```python
from build123d import *

# Parameters (mm, degrees)
SKETCH2_R           = 22.25
SKETCH2_R_2         = 2.5
BOSS_EXTRUDE1_DEPTH = 2.4
SKETCH3_R           = 12.4
BOSS_EXTRUDE2_DEPTH = 47.3
SKETCH4_R           = 3.25
BOSS_EXTRUDE3_DEPTH = 4
SKETCH5_R           = 2.5
BOSS_EXTRUDE4_DEPTH = 8.4
SKETCH6_R           = 12.385
BOSS_EXTRUDE5_DEPTH = 5.1
SKETCH7_R           = 5.9
BOSS_EXTRUDE6_DEPTH = 7.2


with BuildPart() as part:
    # Sketch2 → Boss-Extrude1 (new body)
    with BuildSketch(Plane(origin=(0, 0, 0), x_dir=(1, 0, 0), z_dir=(0, 1, 0))):
        Circle(SKETCH2_R)
        with Locations((0, 17.45)):
            Circle(SKETCH2_R_2, mode=Mode.SUBTRACT)
        with Locations((15.112143296, -8.725)):
            Circle(SKETCH2_R_2, mode=Mode.SUBTRACT)
        with Locations((-15.112143296, -8.725)):
            Circle(SKETCH2_R_2, mode=Mode.SUBTRACT)
    extrude(amount=BOSS_EXTRUDE1_DEPTH)

    # Sketch3 → Boss-Extrude2 (add)
    with BuildSketch(Plane(origin=(0, 2.4, 0), x_dir=(1, 0, 0), z_dir=(0, 1, 0))):
        Circle(SKETCH3_R)
    extrude(amount=BOSS_EXTRUDE2_DEPTH)

    # Sketch4 → Boss-Extrude3 (add)
    with BuildSketch(Plane(origin=(0, 49.7, 0), x_dir=(1, 0, 0), z_dir=(0, 1, 0))):
        Circle(SKETCH4_R)
    extrude(amount=BOSS_EXTRUDE3_DEPTH)

    # Sketch5 → Boss-Extrude4 (add)
    with BuildSketch(Plane(origin=(0, 53.7, 0), x_dir=(1, 0, 0), z_dir=(0, 1, 0))):
        Circle(SKETCH5_R)
    extrude(amount=BOSS_EXTRUDE4_DEPTH)

    # Sketch6 → Boss-Extrude5 (add)
    with BuildSketch(Plane.XZ):
        Circle(SKETCH6_R)
    extrude(amount=BOSS_EXTRUDE5_DEPTH)

    # Sketch7 → Boss-Extrude6 (add)
    with BuildSketch(Plane.XZ.offset(5.1)):
        Circle(SKETCH7_R)
    extrude(amount=BOSS_EXTRUDE6_DEPTH)


solid = part.part
```
Check sheet for the modelled part. Datum: model origin and axes. Units: mm. A direction names the side the tool comes from. Coordinates: 2 decimals unless noted, no trailing zeros. Order: outer loops, then holes, each group sorted by start corner. A loop starts at its lowest first (then second) coordinate and runs counter-clockwise, first axis right, second up. Notation, with made-up numbers: M 68.25,61 L 104.25,61 A29 ccw 104.25,92 Z; hole C -25,53.5 d6. An arc over 180 degrees is marked long. Write each question's results on one line, items separated by ' | '. Start each with the question number.
1. Cross-section at D-D on y = 57. Record the cut outline in (x, z), and give its area (3 significant figures).
2. Access from +Z, -Z, +X, -X, +Y, -Y to the whole of each face (thin tool, end or side, straight path). Record for faces 1 (the face through (-12.73, 1.18, 7.97)), 2 (the face through (-5.894, -8.65, 0.259)), 3 (the face through (3, 49.7, 3)).
3. Go/stop test with flat-tipped pins: P1, Ø10, axis at x = -10, z = 0, coming from the +Y side; P2, Ø3, axis at x = -15, z = -7.5, coming from the -Y side; P3, Ø3, axis at x = -10, y = 18.5, coming from the -Z side. Record where each tip stops, or that it passes through.
4. Material ranges on probe 1 along Z at (x, y) = (0, 1); probe 2 along Y at (x, z) = (-8, 12); probe 3 along Y at (x, z) = (-1.5, -12), recorded low to high.
5. Cross-section at A-A on x = 0. Record the cut outline in (y, z) (3 decimals), and give its area (3 significant figures).
6. Cross-section at B-B on z = 0. Record the cut outline in (x, y) (3 decimals), and give its area (3 significant figures).
7. Cross-section at C-C on z = -17.45. Record the cut outline in (x, y).
8. Mould release check, pull along Z, two halves, no side actions. Record for faces 4 (the face through (-0.5, 1.2, -15)), 5 (the face through (10, 2.4, 10)), 6 (the face through (-2.579, 51.672, 1.978)): +Z half, -Z half, draft (parallel to the pull), parting line (faces both ways), or undercut.
Checks:
1) outline: C 0,0 d5 | area: 19.6 mm²
2) face 1: +Y, -Y | face 2: -Y | face 3: +Y
3) P1: stops at y = 49.7 | P2: stops at y = 0 | P3: stops at z = -9.03
4) probe 1: z = -22.25 to -19.95, -14.95 to 22.25 | probe 2: y = 0 to 2.4 | probe 3: y = -5.1 to 49.7
5) outline: M -12.3,-5.9 L -5.1,-5.9 L -5.1,-12.385 L 0,-12.385 L 0,-14.95 L 2.4,-14.95 L 2.4,-12.4 L 49.7,-12.4 L 49.7,-3.25 L 53.7,-3.25 L 53.7,-2.5 L 62.1,-2.5 L 62.1,2.5 L 53.7,2.5 L 53.7,3.25 L 49.7,3.25 L 49.7,12.4 L 2.4,12.4 L 2.4,22.25 L 0,22.25 L 0,12.385 L -5.1,12.385 L -5.1,5.9 L -12.3,5.9 Z; M 0,-22.25 L 2.4,-22.25 L 2.4,-19.95 L 0,-19.95 Z | area: 1,550 mm²
6) outline: M -22.25,0 L -12.385,0 L -12.385,-5.1 L -5.9,-5.1 L -5.9,-12.3 L 5.9,-12.3 L 5.9,-5.1 L 12.385,-5.1 L 12.385,0 L 22.25,0 L 22.25,2.4 L 12.4,2.4 L 12.4,49.7 L 3.25,49.7 L 3.25,53.7 L 2.5,53.7 L 2.5,62.1 L -2.5,62.1 L -2.5,53.7 L -3.25,53.7 L -3.25,49.7 L -12.4,49.7 L -12.4,2.4 L -22.25,2.4 Z | area: 1,560 mm²
7) outline: M -13.8,0 L -2.5,0 L -2.5,2.4 L -13.8,2.4 Z; M 2.5,0 L 13.8,0 L 13.8,2.4 L 2.5,2.4 Z
8) face 4: undercut | face 5: draft | face 6: parting line
